Model file for the job. Use its own axes, mm. A direction names the side the tool comes from. Round coordinates to 2 decimals unless told otherwise and drop trailing zeros. Write each loop counter-clockwise with the first axis right and the second up, starting at its lowest first coordinate (ties: lowest second). Pieces come first, ordered by that corner, then holes. Notation, with made-up numbers: (34, 23.5) - (73, 23.5) arc R16 ccw to (73, 31.5) - close; hole circle Ø6 at (27, 46.5). An arc over 180 degrees is marked (long way). One line per item, written item: value.
Autodesk Inventor part; units mm, degrees
ref_plane "Work Plane2" through (0, 0, 5) normal (0, 0, -1) x (-1, 0, 0)
ref_plane "YZ Plane" through (0, 0, 0) normal (1, 0, 0) x (0, 1, 0)
ref_plane "XZ Plane" through (0, 0, 0) normal (0, 1, 0) x (-1, 0, 0)
sketch "Sketch1" plane through (0, 0, 0) normal (0, 0, 1) x (1, 0, 0)
  line L0 (0, 0) -> (115, 0)
  line L1 (115, 0) -> (115, 75)
  line L2 (115, 75) -> (0, 75)
  line L3 (0, 75) -> (0, 0)
  dimension "d0" = 115
  dimension "d1" = 75
extrude "Extrusion1" add sketch "Sketch1" along normal blind 40
sketch "Sketch2" plane through (0, 0, 40) normal (0, 0, 1) x (1, 0, 0)
  line L0 (115, 75) -> (0, 75)
  line L1 (115, 0) -> (115, 75)
  line L2 (0, 75) -> (115, 75)
  line L3 (115, 75) -> (115, 55)
  line L4 (115, 55) -> (0, 55)
  line L5 (0, 55) -> (0, 75)
  point P0 (0, 0)
  dimension "d4" = 20
extrude "Extrusion2" cut sketch "Sketch2" against normal blind 5
sketch "Sketch3" plane through (115, 0, 0) normal (1, 0, 0) x (0, 0, -1)
  line L0 (0, 75) -> (-35, 75)
  line L1 (-35, 75) -> (-35, 55)
  line L2 (-35, 55) -> (-40, 55)
  line L3 (-40, 0) -> (-40, 55)
  line L4 (0, 0) -> (-40, 0)
  line L5 (0, 70) -> (-30, 70)
  line L6 (-30, 70) -> (-30, 50)
  line L7 (-30, 50) -> (-35, 50)
  line L8 (-35, 50) -> (-35, 5)
  line L9 (-35, 5) -> (0, 5)
  line L10 (0, 5) -> (0, 70)
  line L11 (0, 0) -> (0, 75)
  dimension "d7" = 5
extrude "Extrusion3" cut sketch "Sketch3" against normal through all contours L10 L9 L8 L7 L6 L5
sketch "Sketch11" plane through (0, 0, 0) normal (0, 0, -1) x (-1, 0, 0)
  line L0 (-120, 70) -> (5, 70)
  line L1 (5, 70) -> (5, 65)
  line L2 (5, 65) -> (-120, 65)
  line L3 (-120, 65) -> (-120, 70)
  line L4 (-115, 70) -> (-115, 75)
  point P0 (0, 0)
  point P1 (0, 70)
  dimension "d42" = 5
  dimension "d43" = 5
  dimension "d44" = 5
extrude "Extrusion11" add sketch "Sketch11" against normal blind 30
ref_plane "Work Plane2" through (0, 0, 5) normal (0, 0, -1) x (-1, 0, 0)
sketch "Sketch12" plane through (0, 0, 5) normal (0, 0, -1) x (-1, 0, 0)
  line L0 (-115, 50) -> (-115, 65)
  line L1 (-115, 5) -> (0, 5)
  line L2 (-115, 65) -> (-70, 65)
  line L3 (-70, 65) -> (-70, 5)
  line L4 (-70, 5) -> (-115, 5)
  line L5 (-115, 5) -> (-115, 65)
  line L6 (-108, 50.5) -> (-77, 50.5) construction
  line L7 (-77, 50.5) -> (-77, 19.5) construction
  line L8 (-77, 19.5) -> (-108, 19.5) construction
  line L9 (-108, 19.5) -> (-108, 50.5) construction
  circle A0 centre (-77, 50.5) radius 1.5
  circle A1 centre (-108, 50.5) radius 1.5
  circle A2 centre (-77, 19.5) radius 1.5
  circle A3 centre (-108, 19.5) radius 1.5
  circle A4 centre (-92.5, 35) radius 3
  point P0 (0, 0)
  point P1 (-5, 5)
  point P2 (-92.5, 50.5)
  point P3 (-92.5, 65)
  point P4 (-108, 35)
  point P5 (-115, 35)
  dimension "d47" = 45
  dimension "d48" = 31
  dimension "d49" = 31
  dimension "d50" = 3
  dimension "d51" = 3
  dimension "d52" = 3
  dimension "d53" = 3
  dimension "d54" = 6
extrude "Extrusion12" add sketch "Sketch12" against normal blind 5
sketch "Sketch13" plane through (0, 0, 5) normal (0, 0, -1) x (-1, 0, 0)
  circle A0 centre (-92.5, 35) radius 3
  circle A1 centre (-92.5, 35) radius 12.5
  point P0 (0, 0)
  dimension "d57" = 25
extrude "Extrusion13" cut sketch "Sketch13" against normal blind 2
sketch "Sketch15" plane through (0, 0, 10) normal (0, 0, 1) x (1, 0, 0)
  circle A0 centre (108, 50.5) radius 1.5
  circle A1 centre (108, 19.5) radius 1.5
  circle A2 centre (77, 50.5) radius 1.5
  circle A3 centre (77, 19.5) radius 1.5
  circle A4 centre (77, 50.5) radius 2
  circle A5 centre (108, 50.5) radius 2
  circle A6 centre (108, 19.5) radius 2
  circle A7 centre (77, 19.5) radius 2
  point P0 (0, 0)
  dimension "d60" = 4
  dimension "d61" = 4
  dimension "d62" = 4
  dimension "d63" = 4
extrude "Extrusion14" cut sketch "Sketch15" along normal through all contours A0 | A1 | A2 | A3 | A4 | A5 | A6 | A7
sketch "Sketch16" plane through (115, 5, 35) normal (0, 0, -1) x (-1, 0, 0)
  circle A0 centre (85, 25) radius 10
  circle A1 centre (85, 25) radius 2.5
  line L0 (115, 45) -> (115, 0)
  line L1 (115, -5) -> (0, -5)
  dimension "d66" = 20
  dimension "d67" = 5
  dimension "d68" = 30
  dimension "d69" = 30
extrude "Extrusion15" add sketch "Sketch16" along normal blind 35
properties part number "FA003" material "ABS Plastic"
1. Band-saw the part on D-D on z = 24. Write the cut outline in (x, y).
Report:
outline: (-5, 65) - (120, 65) - (120, 70) - (115, 70) - (115, 75) - (0, 75) - (0, 70) - (-5, 70) - close; (0, 0) - (115, 0) - (115, 5) - (0, 5) - close; circle Ø20 at (30, 30); hole circle Ø5 at (30, 30)
2. Band-saw the part on B-B on y = 15. Write the cut outline in (x, z), plus the area to 3 significant figures.
Report:
outline: (0, 35) - (115, 35) - (115, 40) - (0, 40) - close; (70, 5) - (115, 5) - (115, 10) - (70, 10) - close
area: 800 mm²
3. Band-saw the part on C-C on x = 108. State how many separate pieces and enclosed holes the cut face has, plus the area to 3 significant figures.
Report:
separate pieces: 4
enclosed holes: 0
area: 1,090 mm²
4. Drop flat-ended pins along their axis: pin 1 (20 mm diameter, centred on x = 97.5, y = 41, fed in from -Z); pin 2 (2 mm diameter, centred on y = 42, z = 9.5, fed in from -X); pin 3 (2.5 mm diameter, centred on x = 77, y = 19.5, fed in from +Z); pin 4 (2.5 mm diameter, centred on x = 117, z = 11, fed in from +Y). Give the stop position or say it passes through.
Report:
pin 1: z = 5
pin 2: x = 70
pin 3: through
pin 4: y = 70
5. Band-saw the part on A-A on z = 32.5. Write the cut outline in (x, y).
Report:
outline: (0, 0) - (115, 0) - (115, 5) - (0, 5) - close; (0, 50) - (75.06, 50) arc R2 cw (long way) to (78.94, 50) - (106.06, 50) arc R2 cw (long way) to (109.94, 50) - (115, 50) - (115, 75) - (0, 75) - close; circle Ø20 at (30, 30); hole circle Ø5 at (30, 30)
6. Mould opens along Y. For faces 1 (the face through (95.5, 35.1, 8.5)), 2 (the face through (58, 55, 38)), 3 (the face through (57, 65, 35)) say: released by +Y, released by -Y, zero draft, split by the parting line, or undercut.
Report:
face 1: undercut
face 2: released by +Y
face 3: zero draft
7. Wall check: probe 1 along Y at (x, z) = (30, 10); probe 2 along Y at (x, z) = (77, 37.9); probe 3 along Z at (x, y) = (93, 57). Give the ranges that are in metal, low to high. Write a range as [from, to].
Report:
probe 1: [0, 5], [20, 27.5], [32.5, 40], [65, 75]
probe 2: [0, 17.5], [21.5, 48.5], [52.5, 55]
probe 3: [5, 10], [30, 35]
8. Tool access for faces 4 (the face through (-2, 68, 30)), 5 (the face through (107.566, 52.452, 36.041)), 6 (the face through (76.31, 49.17, 7.46)), 7 (the face through (58, 70, 0)), 8 (the face through (90, 32, 7)): list every direction of +Z, -Z, +X, -X, +Y, -Y with a clear straight run to the whole face (end or side of a thin tool).
Report:
face 4: +Z, -X, +Y, -Y
face 5: +Z
face 6: +Z, -Z
face 7: -Z, +X, -X, +Y, -Y
face 8: -Z
